Build history of the part. All positions in model axes, mm. A direction names the side the tool comes from. Give positions to 0.01 mm unless a question says otherwise; leave off trailing zeros. Write item = value, one per line. Start each with the question number.
Q1. Drop flat-ended pins along their axis: P1, Ø3, axis at y = 4.5, z = 10.5, coming from the -X side; P2, Ø1.5, axis at x = 20, y = 4.5, coming from the -Z side; P3, Ø1.6, axis at x = 0.5, y = 2.5, coming from the +Z side. Give the stop position or say it passes through.
Q2. Wall check: line 1 (X direction, y = 2.4, z = 76); line 2 (Z direction, x = -21, y = 1.5); line 3 (Z direction, x = 40.5, y = 3.55). Give the ranges that are in metal, low to high.
Q3. Mould opens along X. For faces 1 (the face through (31.691, 1.233, 84.236)), 2 (the face through (1, 5.5, -1)), 3 (the face through (-88.528, 0.986, -0.796)) say: pulls with the +X half, pulls with the -X half, needs draft (parallel to the pull), parting line crosses it, or undercut.
Q4. Saw through at A-A, the plane x = 0. Give the number of separate pieces and of enclosed holes in the cut face, then the cut area to 3 significant figures.
Q5. Tool access for faces 4 (the face through (-4.99, 3.33, 79.8)), 5 (the face through (79.884, 3.774, -0.193)), 6 (the face through (1, 0, -1)): list every direction of +Z, -Z, +X, -X, +Y, -Y with a clear straight run to the whole face (end or side of a thin tool).
from build123d import *

# Parameters (mm, degrees)
SKETCH1_R                                    = 90
BOSS_EXTRUDE1_DEPTH                          = 5.5
CBORE_FOR_M5_HEX_HEAD_CAP_SCREW1_D           = 5.3
CBORE_FOR_M5_HEX_HEAD_CAP_SCREW1_DEPTH       = 6
CBORE_FOR_M5_HEX_HEAD_CAP_SCREW1_CBORE_D     = 12.238
CBORE_FOR_M5_HEX_HEAD_CAP_SCREW1_CBORE_DEPTH = 3.5
CBORE_FOR_M5_HEX_HEAD_CAP_SCREW1_TIP         = 1.59228064
FILLET1_R                                    = 3
CUT_EXTRUDE1_DEPTH                           = 31
CUT_REVOLVE_THIN8_START                      = 70.039018211
CUT_REVOLVE_THIN8_DEPTH                      = 19.960981889


# Read off the part's stored shape, not the designer's step: Cut-Revolve-Thin8
with BuildPart() as part:
    # Sketch1 → Boss-Extrude1 (new body)
    with BuildSketch(Plane(origin=(0, 0, 0), x_dir=(1, 0, 0), z_dir=(0, 1, 0))):
        with Locations(Location((0, 0, 0), (0, 0, 270))):
            Circle(SKETCH1_R)
    extrude(amount=BOSS_EXTRUDE1_DEPTH)

    # CBORE for M5 Hex Head Cap Screw1
    with Locations(Plane(origin=(0, 5.5, 0), x_dir=(1, 0, 0), z_dir=(0, 1, 0))):
        with Locations((0, 86), (-86, 0), (86, 0)):
            CounterBoreHole(CBORE_FOR_M5_HEX_HEAD_CAP_SCREW1_D / 2, CBORE_FOR_M5_HEX_HEAD_CAP_SCREW1_CBORE_D / 2, CBORE_FOR_M5_HEX_HEAD_CAP_SCREW1_CBORE_DEPTH, depth=CBORE_FOR_M5_HEX_HEAD_CAP_SCREW1_DEPTH)
            with Locations((0, 0, -(CBORE_FOR_M5_HEX_HEAD_CAP_SCREW1_DEPTH + CBORE_FOR_M5_HEX_HEAD_CAP_SCREW1_TIP / 2))):  # 118° drill point
                Cone(0, CBORE_FOR_M5_HEX_HEAD_CAP_SCREW1_D / 2, CBORE_FOR_M5_HEX_HEAD_CAP_SCREW1_TIP, mode=Mode.SUBTRACT)

    # Fillet1
    fillet1_edges = [part.edges().sort_by_distance(p)[0] for p in [
        (-61.942775174, 5.5, 65.292362523),
        (-63.639610307, 5.5, -63.639610307),
        (63.639610307, 5.5, -63.639610307),
    ]]
    fillet(fillet1_edges, radius=FILLET1_R)

    # Sketch5 → Cut-Extrude1 (cut)
    with BuildSketch(Plane(origin=(0, 5.5, 0), x_dir=(1, 0, 0), z_dir=(0, 1, 0))):
        with BuildLine():
            add(Edge.make_bspline(
                [(-3.285569008, 57.868614525), (-3.024078757, 58.587053083), (-2.783851066, 59.272048996), (-2.563116696, 59.924191453)],
                knots=[0, 0, 0, 0, 0.04164671, 0.04164671, 0.04164671, 0.04164671], degree=3))
            ThreePointArc((-3.285569008, 57.868614525), (0, 54.583045517), (3.285569008, 57.868614525))
            add(Edge.make_bspline(
                [(2.563054058, 59.924269555), (2.783803493, 59.272145294), (3.0240518, 58.587127147), (3.285569008, 57.868614525)],
                knots=[0.958431192, 0.958431192, 0.958431192, 0.958431192, 1, 1, 1, 1], degree=3))
            ThreePointArc((2.563054058, 59.924269555), (-5.0059e-05, 61.154183532), (-2.563116696, 59.924191453))
        make_face()
        with BuildLine():
            ThreePointArc((-2.563116696, 59.924191453), (-3.099698411, 58.958033389), (-3.285569008, 57.868614525))
            add(Edge.make_bspline(
                [(-3.285569008, 57.868614525), (-3.024078757, 58.587053083), (-2.783851066, 59.272048996), (-2.563116696, 59.924191453)],
                knots=[0, 0, 0, 0, 0.04164671, 0.04164671, 0.04164671, 0.04164671], degree=3))
        make_face()
        with BuildLine():
            add(Edge.make_bspline(
                [(2.563054058, 59.924269555), (2.783803493, 59.272145294), (3.0240518, 58.587127147), (3.285569008, 57.868614525)],
                knots=[0.958431192, 0.958431192, 0.958431192, 0.958431192, 1, 1, 1, 1], degree=3))
            ThreePointArc((3.285569008, 57.868614525), (3.099681813, 58.958080616), (2.563054058, 59.924269555))
        make_face()
        with BuildLine():
            add(Edge.make_bspline(
                [(-2.563116696, 59.924191453), (-0.133769336, 67.101508499), (0.002619877, 73.497835408), (0.128574166, 67.116058723), (2.563054058, 59.924269555)],
                knots=[0.04164671, 0.04164671, 0.04164671, 0.04164671, 0.5, 0.958431192, 0.958431192, 0.958431192, 0.958431192], degree=3))
            ThreePointArc((-2.563116696, 59.924191453), (-5.0059e-05, 61.154183532), (2.563054058, 59.924269555))
        make_face()
    extrude(amount=-CUT_EXTRUDE1_DEPTH, mode=Mode.SUBTRACT)

    # Cut-Revolve-Thin8 outline → Cut-Revolve-Thin8 (cut)
    with BuildSketch(Plane.XY.offset(CUT_REVOLVE_THIN8_START)):
        with BuildLine():
            Line((-6, 0), (6, 0))
            ThreePointArc((6, 0), (5.019337335, 3.287286528), (2.397915762, 5.5))
            Line((2.397915762, 5.5), (-2.397915762, 5.5))
            ThreePointArc((-2.397915762, 5.5), (-5.019337335, 3.287286528), (-6, 0))
        make_face()
    extrude(amount=CUT_REVOLVE_THIN8_DEPTH, mode=Mode.SUBTRACT)


solid = part.part
Report:
q1.P1 = -89.39
q1.P2 = -87.51
q1.P3 = 70.04
q2.line_1 = -48.21 to -5.5, 5.5 to 48.21
q2.line_2 = -87.52 to 87.52
q2.line_3 = -80.16 to 80.16
q3.face_1 = parting line crosses it
q3.face_2 = needs draft
q3.face_3 = undercut
q4.separate_pieces = 3
q4.enclosed_holes = 0
q4.area = 748 mm2
q5.face_4 = +Z, -Y
q5.face_5 = +Y
q5.face_6 = +Z, -Z, +X, -X, -Y
